Build history of the part. All positions in model axes, mm. A direction names the side the tool comes from. Round coordinates to 2 decimals unless told otherwise and drop trailing zeros. Order: outer loops, then holes, each group sorted by start corner. A loop starts at its lowest first (then second) coordinate and runs counter-clockwise, first axis right, second up. Notation, with made-up numbers: (24.25, 21) -> (60.25, 21) arc R11 cw to (60.25, 42) -> close; hole circle Ø4 at (50, 85). An arc over 180 degrees is marked (long way). Answer as a JSON object with one key per item and string values.
from build123d import *

# Parameters (mm, degrees)
F1_DEPTH     = 20
F3_D         = 5
F5_T1_DEPTH  = 150
F5_T3_DEPTH  = 40
F5_T5_DEPTH  = 30
F5_T7_DEPTH  = 25
F5_T9_DEPTH  = 100
F5_T11_DEPTH = 30
F5_T25_DEPTH = 105
F5_T29_DEPTH = 30
F5_T36_DEPTH = 30
F5_T40_DEPTH = 105
F5_T47_DEPTH = 30
F5_T51_DEPTH = 105
F5_T58_DEPTH = 105
F5_T62_DEPTH = 30


# Not quite as in the source:
# - a fillet or chamfer that OpenCascade refuses, or shapes differently, is made with other operations: its cross-section is extruded or revolved along the edge and cut away or added


with BuildPart() as f1:
    # F0 (on Top) → F1 (new body)
    with BuildSketch(Plane.XY):
        Polygon((70, 30), (0, 30), (0, 20), (50, 20), (50, 0), (70, 0), align=None)
    extrude(amount=F1_DEPTH)

    # F3 (through all)
    with Locations(Plane(origin=(0, 0, 0), x_dir=(1, 0, 0), z_dir=(0, 0, -1))):
        with Locations((65, -7.3669357225)):
            Hole(F3_D / 2)

    # F4: F1 across face


with BuildPart() as f1_1:
    add(f1.part)
    add(f1.part.mirror(Plane(origin=(0, 25, 10), x_dir=(0, -1, 0), z_dir=(-1, 0, 0))))

    # F5: fillet of radius 2 on 20 edges, made by hand

    # F5_s2 → F5_t1 (cut)
    with BuildSketch(Plane.YZ.offset(-75)):
        with BuildLine():
            ThreePointArc((30, 18), (29.4142135624, 19.4142135624), (28, 20))
            Line((28, 20), (30, 20))
            Line((30, 20), (30, 18))
        make_face()
        with BuildLine():
            ThreePointArc((30, 2), (29.4142135624, 0.5857864376), (28, 0))
            Line((28, 0), (30, 0))
            Line((30, 0), (30, 2))
        make_face()
    extrude(amount=F5_T1_DEPTH, mode=Mode.SUBTRACT)

    # F5_s4 → F5_t3 (cut)
    with BuildSketch(Plane.XZ.offset(-35)):
        with BuildLine():
            ThreePointArc((-70, 18), (-69.4142135624, 19.4142135624), (-68, 20))
            Line((-68, 20), (-70, 20))
            Line((-70, 20), (-70, 18))
        make_face()
        with BuildLine():
            ThreePointArc((68, 20), (69.4142135624, 19.4142135624), (70, 18))
            Line((70, 18), (70, 20))
            Line((70, 20), (68, 20))
        make_face()
        with BuildLine():
            ThreePointArc((-68, 0), (-69.4142135624, 0.5857864376), (-70, 2))
            Line((-70, 2), (-70, 0))
            Line((-70, 0), (-68, 0))
        make_face()
        with BuildLine():
            ThreePointArc((68, 0), (69.4142135624, 0.5857864376), (70, 2))
            Line((70, 2), (70, 0))
            Line((70, 0), (68, 0))
        make_face()
    extrude(amount=F5_T3_DEPTH, mode=Mode.SUBTRACT)

    # F5_s6 → F5_t5 (cut)
    with BuildSketch(Plane.YZ.offset(-75)):
        with BuildLine():
            ThreePointArc((0, 18), (0.5857864376, 19.4142135624), (2, 20))
            Line((2, 20), (0, 20))
            Line((0, 20), (0, 18))
        make_face()
        with BuildLine():
            ThreePointArc((2, 0), (0.5857864376, 0.5857864376), (0, 2))
            Line((0, 2), (0, 0))
            Line((0, 0), (2, 0))
        make_face()
    extrude(amount=F5_T5_DEPTH, mode=Mode.SUBTRACT)

    # F5_s8 → F5_t7 (cut)
    with BuildSketch(Plane.XZ.offset(-20)):
        with BuildLine():
            ThreePointArc((-50, 18), (-50.5857864376, 19.4142135624), (-52, 20))
            Line((-52, 20), (-50, 20))
            Line((-50, 20), (-50, 18))
        make_face()
        with BuildLine():
            ThreePointArc((50, 18), (50.5857864376, 19.4142135624), (52, 20))
            Line((52, 20), (50, 20))
            Line((50, 20), (50, 18))
        make_face()
        with BuildLine():
            ThreePointArc((-52, 0), (-50.5857864376, 0.5857864376), (-50, 2))
            Line((-50, 2), (-50, 0))
            Line((-50, 0), (-52, 0))
        make_face()
        with BuildLine():
            ThreePointArc((52, 0), (50.5857864376, 0.5857864376), (50, 2))
            Line((50, 2), (50, 0))
            Line((50, 0), (52, 0))
        make_face()
    extrude(amount=F5_T7_DEPTH, mode=Mode.SUBTRACT)

    # F5_s10 → F5_t9 (cut)
    with BuildSketch(Plane.YZ.offset(-50)):
        with BuildLine():
            ThreePointArc((20, 18), (20.5857864376, 19.4142135624), (22, 20))
            Line((22, 20), (20, 20))
            Line((20, 20), (20, 18))
        make_face()
        with BuildLine():
            ThreePointArc((22, 0), (20.5857864376, 0.5857864376), (20, 2))
            Line((20, 2), (20, 0))
            Line((20, 0), (22, 0))
        make_face()
    extrude(amount=F5_T9_DEPTH, mode=Mode.SUBTRACT)

    # F5_s12 → F5_t11 (cut)
    with BuildSketch(Plane.YZ.offset(45)):
        with BuildLine():
            ThreePointArc((0, 18), (0.5857864376, 19.4142135624), (2, 20))
            Line((2, 20), (0, 20))
            Line((0, 20), (0, 18))
        make_face()
        with BuildLine():
            ThreePointArc((2, 0), (0.5857864376, 0.5857864376), (0, 2))
            Line((0, 2), (0, 0))
            Line((0, 0), (2, 0))
        make_face()
    extrude(amount=F5_T11_DEPTH, mode=Mode.SUBTRACT)

    # F5_s13 → F5_t14 (revolve, cut)
    with BuildSketch(Plane.XZ.offset(-7.3669357225)):
        with BuildLine():
            ThreePointArc((67.5, 18), (68.0857864376, 19.4142135624), (69.5, 20))
            Line((69.5, 20), (67.5, 20))
            Line((67.5, 20), (67.5, 18))
        make_face()
    revolve(axis=Axis((65, 7.3669357225, 20), (0, 0, -1)), mode=Mode.SUBTRACT)

    # F5_s15 → F5_t16 (revolve, cut)
    with BuildSketch(Plane.XZ.offset(-7.3669357225)):
        with BuildLine():
            ThreePointArc((-67.5, 18), (-68.0857864376, 19.4142135624), (-69.5, 20))
            Line((-69.5, 20), (-67.5, 20))
            Line((-67.5, 20), (-67.5, 18))
        make_face()
    revolve(axis=Axis((-65, 7.3669357225, 20), (0, 0, 1)), mode=Mode.SUBTRACT)

    # F5_s17 → F5_t18 (revolve, cut)
    with BuildSketch(Plane.XZ.offset(-7.3669357225)):
        with BuildLine():
            ThreePointArc((69.5, 0), (68.0857864376, 0.5857864376), (67.5, 2))
            Line((67.5, 2), (67.5, 0))
            Line((67.5, 0), (69.5, 0))
        make_face()
    revolve(axis=Axis((65, 7.3669357225, 0), (0, 0, -1)), mode=Mode.SUBTRACT)

    # F5_s19 → F5_t20 (revolve, cut)
    with BuildSketch(Plane.XZ.offset(-7.3669357225)):
        with BuildLine():
            ThreePointArc((-69.5, 0), (-68.0857864376, 0.5857864376), (-67.5, 2))
            Line((-67.5, 2), (-67.5, 0))
            Line((-67.5, 0), (-69.5, 0))
        make_face()
    revolve(axis=Axis((-65, 7.3669357225, 0), (0, 0, 1)), mode=Mode.SUBTRACT)


with BuildPart() as f5_tool23:
    # F5_s24 → F5_t25 (new body)
    with BuildSketch(Plane.YZ.offset(-55)):
        with BuildLine():
            ThreePointArc((20, 18), (20.5857864376, 19.4142135624), (22, 20))
            Line((22, 20), (20, 20))
            Line((20, 20), (20, 18))
        make_face()
    extrude(amount=F5_T25_DEPTH)

    split(bisect_by=Plane.YZ.offset(-50), keep=Keep.BOTTOM)


with BuildPart() as f5_tool27:
    # F5_s28 → F5_t29 (new body)
    with BuildSketch(Plane.XZ.offset(-25)):
        with BuildLine():
            ThreePointArc((-50, 18), (-50.5857864376, 19.4142135624), (-52, 20))
            Line((-52, 20), (-50, 20))
            Line((-50, 20), (-50, 18))
        make_face()
    extrude(amount=F5_T29_DEPTH)

    split(bisect_by=Plane.XZ.offset(-20), keep=Keep.BOTTOM)


with BuildPart() as f5_tool23_1:
    add(f5_tool23.part)

    # F5_t31: intersect F5_tool27
    add(f5_tool27.part, mode=Mode.INTERSECT)


with BuildPart() as f1_2:
    add(f1_1.part)

    # F5_t21: cut F5_tool23
    add(f5_tool23_1.part, mode=Mode.SUBTRACT)


with BuildPart() as f5_tool34:
    # F5_s35 → F5_t36 (new body)
    with BuildSketch(Plane.XZ.offset(-25)):
        with BuildLine():
            ThreePointArc((50, 18), (50.5857864376, 19.4142135624), (52, 20))
            Line((52, 20), (50, 20))
            Line((50, 20), (50, 18))
        make_face()
    extrude(amount=F5_T36_DEPTH)

    split(bisect_by=Plane.XZ.offset(-20), keep=Keep.BOTTOM)


with BuildPart() as f5_tool38:
    # F5_s39 → F5_t40 (new body)
    with BuildSketch(Plane.YZ.offset(-50)):
        with BuildLine():
            ThreePointArc((20, 18), (20.5857864376, 19.4142135624), (22, 20))
            Line((22, 20), (20, 20))
            Line((20, 20), (20, 18))
        make_face()
    extrude(amount=F5_T40_DEPTH)

    split(bisect_by=Plane.YZ.offset(50), keep=Keep.TOP)


with BuildPart() as f5_tool34_1:
    add(f5_tool34.part)

    # F5_t42: intersect F5_tool38
    add(f5_tool38.part, mode=Mode.INTERSECT)


with BuildPart() as f1_3:
    add(f1_2.part)

    # F5_t32: cut F5_tool34
    add(f5_tool34_1.part, mode=Mode.SUBTRACT)


with BuildPart() as f5_tool45:
    # F5_s46 → F5_t47 (new body)
    with BuildSketch(Plane.XZ.offset(-25)):
        with BuildLine():
            ThreePointArc((-52, 0), (-50.5857864376, 0.5857864376), (-50, 2))
            Line((-50, 2), (-50, 0))
            Line((-50, 0), (-52, 0))
        make_face()
    extrude(amount=F5_T47_DEPTH)

    split(bisect_by=Plane.XZ.offset(-20), keep=Keep.BOTTOM)


with BuildPart() as f5_tool49:
    # F5_s50 → F5_t51 (new body)
    with BuildSketch(Plane.YZ.offset(50)):
        with BuildLine():
            ThreePointArc((22, 0), (20.5857864376, 0.5857864376), (20, 2))
            Line((20, 2), (20, 0))
            Line((20, 0), (22, 0))
        make_face()
    extrude(amount=-F5_T51_DEPTH)

    split(bisect_by=Plane.YZ.offset(-50), keep=Keep.BOTTOM)


with BuildPart() as f5_tool45_1:
    add(f5_tool45.part)

    # F5_t53: intersect F5_tool49
    add(f5_tool49.part, mode=Mode.INTERSECT)


with BuildPart() as f1_4:
    add(f1_3.part)

    # F5_t43: cut F5_tool45
    add(f5_tool45_1.part, mode=Mode.SUBTRACT)


with BuildPart() as f5_tool56:
    # F5_s57 → F5_t58 (new body)
    with BuildSketch(Plane.YZ.offset(55)):
        with BuildLine():
            ThreePointArc((22, 0), (20.5857864376, 0.5857864376), (20, 2))
            Line((20, 2), (20, 0))
            Line((20, 0), (22, 0))
        make_face()
    extrude(amount=-F5_T58_DEPTH)

    split(bisect_by=Plane.YZ.offset(50), keep=Keep.TOP)


with BuildPart() as f5_tool60:
    # F5_s61 → F5_t62 (new body)
    with BuildSketch(Plane.XZ.offset(-25)):
        with BuildLine():
            ThreePointArc((52, 0), (50.5857864376, 0.5857864376), (50, 2))
            Line((50, 2), (50, 0))
            Line((50, 0), (52, 0))
        make_face()
    extrude(amount=F5_T62_DEPTH)

    split(bisect_by=Plane.XZ.offset(-20), keep=Keep.BOTTOM)


with BuildPart() as f5_tool56_1:
    add(f5_tool56.part)

    # F5_t64: intersect F5_tool60
    add(f5_tool60.part, mode=Mode.INTERSECT)


with BuildPart() as f1_5:
    add(f1_4.part)

    # F5_t54: cut F5_tool56
    add(f5_tool56_1.part, mode=Mode.SUBTRACT)


solid = f1_5.part
1) Which spindle directions (+Z, -Z, +X, -X, +Y, -Y) get a long thin tool onto all of the face, cutting with end or side? Do faces 5 (the face through (-60, 0, 10)), 6 (the face through (-50, 10, 10)). Say none if no direction does.
Checked values:
{"face 5": "+Z, -Z, +X, -X, -Y", "face 6": "+Z, -Z, -Y"}
2) Flat gauge pins, fed straight in: pin 1 Ø5 at (x, y) = (-24, 20) entering from -Z; pin 2 Ø6 at (x, y) = (65, 7.37) entering from +Z. Where does each tip first touch, or does it go through?
Checked values:
{"pin 1": "stops at z = 0", "pin 2": "stops at z = 19.33"}
3) Pull direction X, two halves, no side cores. Call faces 1 (the face through (60, 0, 10)), 2 (the face through (-70, 15, 10)), 3 (the face through (-62.615, 6.616, 10.112)), 4 (the face through (50, 10, 10)): pulls with the +X half, pulls with the -X half, needs draft (parallel to the pull), parting line crosses it, or undercut.
Checked values:
{"face 1": "needs draft", "face 2": "pulls with the -X half", "face 3": "undercut", "face 4": "undercut"}
4) Cut at A-A, the plane x = 65. Give the cut face in (y, z).
Checked values:
{"outline": "(0, 2) arc R2 ccw to (2, 0) -> (2.87, 0) arc R2 ccw to (4.87, 2) -> (4.87, 18) arc R2 ccw to (2.87, 20) -> (2, 20) arc R2 ccw to (0, 18) -> close; (9.87, 2) arc R2 ccw to (11.87, 0) -> (28, 0) arc R2 ccw to (30, 2) -> (30, 18) arc R2 ccw to (28, 20) -> (11.87, 20) arc R2 ccw to (9.87, 18) -> close"}
5) Cut at C-C, the plane z = 11.5. Give the cut face in (x, y).
Checked values:
{"outline": "(-70, 0) -> (-50, 0) -> (-50, 20) -> (50, 20) -> (50, 0) -> (70, 0) -> (70, 30) -> (-70, 30) -> close; hole circle Ø5 at (-65, 7.37); hole circle Ø5 at (65, 7.37)"}
6) Probe L1, parallel to X at y = 16, z = 14.75; L2, parallel to Y at x = -65, z = 10.75; L3, parallel to X at y = 9.5, z = 3.25. List the from-to ranges inside material, lowest first. Write a range as from..to.
Checked values:
{"L1": "x = -70..-50, 50..70", "L2": "y = 0..4.87, 9.87..30", "L3": "x = -70..-66.3, -63.7..-50, 50..63.7, 66.3..70"}
7) Cut at B-B, the plane x = 27.5. Give the cut face in (y, z), plus the area to 3 significant figures.
Checked values:
{"outline": "(20, 2) arc R2 ccw to (22, 0) -> (28, 0) arc R2 ccw to (30, 2) -> (30, 18) arc R2 ccw to (28, 20) -> (22, 20) arc R2 ccw to (20, 18) -> close", "area": "197 mm²"}
